from build123d import *

# Parameters (mm, degrees)
CROQUIS1_R              = 31.5
CROQUIS1_R_2            = 1.5
CROQUIS1_R_3            = 2
SALIENTE_EXTRUIR1_DEPTH = 3
CORTAR_EXTRUIR2_DEPTH   = 1.5
CROQUIS4_W              = 15
CROQUIS4_H              = 25
SALIENTE_EXTRUIR2_DEPTH = 3
SALIENTE_EXTRUIR3_DEPTH = 25
CORTAR_EXTRUIR3_DEPTH   = 23
SALIENTE_EXTRUIR4_DEPTH = 5
CORTAR_EXTRUIR4_DEPTH   = 2


with BuildPart() as part:
    # Croquis1 → Saliente-Extruir1 (new body)
    with BuildSketch(Plane.XY):
        with Locations((-43.449193048, 8.207110309)):
            Circle(CROQUIS1_R)
        with Locations((-60.066202406, 24.824119667)):
            Circle(CROQUIS1_R_2, mode=Mode.SUBTRACT)
        with Locations((-26.83218369, 24.824119667)):
            Circle(CROQUIS1_R_2, mode=Mode.SUBTRACT)
        with Locations((-26.83218369, -8.409899049)):
            Circle(CROQUIS1_R_2, mode=Mode.SUBTRACT)
        with Locations((-60.066202406, -8.409899049)):
            Circle(CROQUIS1_R_2, mode=Mode.SUBTRACT)
        with Locations((-43.449193048, 8.207110309)):
            Circle(CROQUIS1_R_3, mode=Mode.SUBTRACT)
    extrude(amount=SALIENTE_EXTRUIR1_DEPTH)

    # Croquis3 → Cortar-Extruir2 (cut)
    with BuildSketch(Plane.XY.offset(3)):
        with BuildLine():
            Line((-41.199193048, 22.957110309), (-40.349193048, 10.457110309))
            Line((-40.349193048, 10.457110309), (-36.699193048, 10.457110309))
            ThreePointArc((-36.699193048, 10.457110309), (-34.449193048, 8.207110309), (-36.699193048, 5.957110309))
            Line((-36.699193048, 5.957110309), (-39.699193048, 5.957110309))
            Line((-39.699193048, 5.957110309), (-41.199193048, -8.542889691))
            ThreePointArc((-41.199193048, -8.542889691), (-43.449193048, -10.792889691), (-45.699193048, -8.542889691))
            Line((-45.699193048, -8.542889691), (-47.199193048, 5.957110309))
            Line((-47.199193048, 5.957110309), (-50.199193048, 5.957110309))
            ThreePointArc((-50.199193048, 5.957110309), (-52.449193048, 8.207110309), (-50.199193048, 10.457110309))
            Line((-50.199193048, 10.457110309), (-46.549193048, 10.457110309))
            Line((-46.549193048, 10.457110309), (-45.699193048, 22.957110309))
            ThreePointArc((-45.699193048, 22.957110309), (-43.449193048, 25.207110309), (-41.199193048, 22.957110309))
        make_face()
    extrude(amount=-CORTAR_EXTRUIR2_DEPTH, mode=Mode.SUBTRACT)

    # Croquis4 → Saliente-Extruir2 (add)
    with BuildSketch(Plane(origin=(0, 0, 0), x_dir=(-1, 0, 0), z_dir=(0, 0, -1))):
        with Locations((43.449193048, 8.207110309)):
            Rectangle(CROQUIS4_W, CROQUIS4_H)
    extrude(amount=SALIENTE_EXTRUIR2_DEPTH)

    # Croquis5 → Saliente-Extruir3 (add)
    with BuildSketch(Plane.XZ.offset(4.292889691)):
        Polygon((-35.949193048, 0), (-32.949193048, 0), (-35.949193048, -3), align=None)
        Polygon((-50.949193048, 0), (-53.949193048, 0), (-50.949193048, -3), align=None)
    extrude(amount=-SALIENTE_EXTRUIR3_DEPTH)

    # Croquis6 → Cortar-Extruir3 (cut)
    with BuildSketch(Plane.XZ.offset(4.292889691)):
        Polygon((-35.949193048, 0), (-50.949193048, 0), (-47.949193048, -3), (-38.949193048, -3), align=None)
    extrude(amount=-CORTAR_EXTRUIR3_DEPTH, mode=Mode.SUBTRACT)

    # Croquis7 → Saliente-Extruir4 (add)
    with BuildSketch(Plane.XZ.offset(4.292889691)):
        Polygon((-39.149193048, -3), (-36.649193048, -0.5), (-36.249193048, -0.5), (-38.749193048, -3), align=None)
        Polygon((-50.249193048, -0.5), (-50.649193048, -0.5), (-48.149193048, -3), (-47.749193048, -3), align=None)
    extrude(amount=SALIENTE_EXTRUIR4_DEPTH)

    # Croquis8 → Cortar-Extruir4 (cut)
    with BuildSketch(Plane(origin=(0, 0, 0), x_dir=(-1, 0, 0), z_dir=(0, 0, -1))):
        Polygon((30.296285305, 24.824119667), (28.564234497, 27.824119667), (25.100132882, 27.824119667), (23.368082075, 24.824119667), (25.100132882, 21.824119667), (28.564234497, 21.824119667), align=None)
        Polygon((63.530304021, 24.824119667), (61.798253213, 27.824119667), (58.334151598, 27.824119667), (56.60210079, 24.824119667), (58.334151598, 21.824119667), (61.798253213, 21.824119667), align=None)
        Polygon((30.296285305, -8.409899049), (28.564234497, -5.409899049), (25.100132882, -5.409899049), (23.368082075, -8.409899049), (25.100132882, -11.409899049), (28.564234497, -11.409899049), align=None)
        Polygon((63.530304021, -8.409899049), (61.798253213, -5.409899049), (58.334151598, -5.409899049), (56.60210079, -8.409899049), (58.334151598, -11.409899049), (61.798253213, -11.409899049), align=None)
    extrude(amount=-CORTAR_EXTRUIR4_DEPTH, mode=Mode.SUBTRACT)


solid = part.part
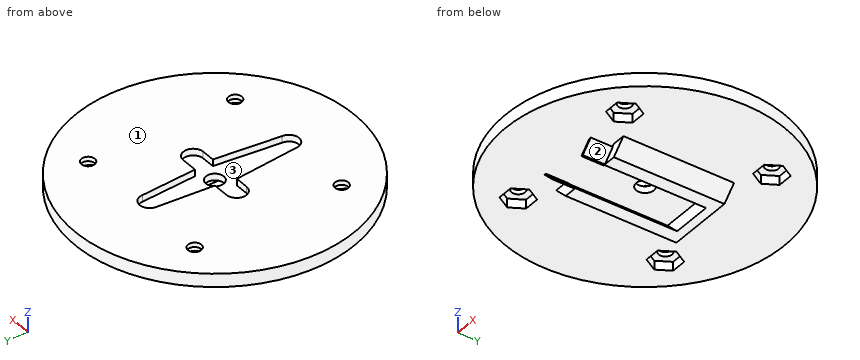
Input: part model. Units: mm. Frame: model coordinates. Face numbers are marked on the shaded views. Give positions to 0.01 mm unless a question says otherwise; leave off trailing zeros. Write each loop counter-clockwise with the first axis right and the second up, starting at its lowest first coordinate (ties: lowest second). Pieces come first, ordered by that corner, then holes. Notation, with made-up numbers: M -20.5,-29 L 28.5,-29 A19 ccw 28.5,-4 Z; hole C -28,54 d2. An arc over 180 degrees is marked long. Write item = value, one per line. Start each with the question number.
1) Cut plane A-A on y = 9. Return the cut outline in (x, z).
2) Cut plane B-B on z = 0.75. Return the cut outline in (x, y), then the cut area to 3 significant figures.
3) Cut plane C-C on x = -44. Return the cut outline in (y, z).
4) Cut plane D-D on y = -0.5. Return the cut outline in (x, z).
5) Draft query along X for the marked faces 1, 2 and 3. Return one class per face: +X half, -X half, draft (parallel to the pull), parting line (faces both ways), or undercut.
6) Material intervals for line 1 along Y through (x, z) = (-24, 0.5); line 2 along X through (y, z) = (23.5, 2.1); line 3 along X through (y, z) = (23, 0.4), sorted ascending. Write a range as [from, to].
7) First-contact query: pin 1 Ø2 at (x, z) = (-33.5, 0) entering from -Y; pin 2 Ø1 at (y, z) = (-10.5, 0.5) entering from -X; pin 3 Ø2 at (x, z) = (-60, 1) entering from -Y; pin 4 Ø2.5 at (x, y) = (-43.45, 8.21) entering from +Z. Flat tips, straight axial feed; report the tip coordinate or a pass-through.
Solved:
q1.outline = M -74.94,0 L -53.95,0 L -50.95,-3 L -47.95,-3 L -50.95,0 L -45.29,0 L -45.29,1.5 L -52.3,1.5 L -52.3,3 L -74.94,3 Z; M -41.61,0 L -35.95,0 L -38.95,-3 L -35.95,-3 L -32.95,0 L -11.96,0 L -11.96,3 L -34.59,3 L -34.59,1.5 L -41.61,1.5 Z
q2.outline = C -43.45,8.21 d63; hole M -63.53,-8.41 L -61.8,-11.41 L -58.33,-11.41 L -56.6,-8.41 L -58.33,-5.41 L -61.8,-5.41 Z; hole M -63.53,24.82 L -61.8,21.82 L -58.33,21.82 L -56.6,24.82 L -58.33,27.82 L -61.8,27.82 Z; hole C -43.45,8.21 d4; hole M -30.3,-8.41 L -28.56,-11.41 L -25.1,-11.41 L -23.37,-8.41 L -25.1,-5.41 L -28.56,-5.41 Z; hole M -30.3,24.82 L -28.56,21.82 L -25.1,21.82 L -23.37,24.82 L -25.1,27.82 L -28.56,27.82 Z
q2.area = 2,980 mm2
q3.outline = M -23.29,0 L 6.28,0 L 6.28,1.5 L -10.72,1.5 L -10.72,3 L -23.29,3 Z; M 10.13,0 L 18.71,0 L 18.71,-3 L 20.71,-3 L 20.71,0 L 39.7,0 L 39.7,3 L 25.14,3 L 25.14,1.5 L 10.13,1.5 Z
q4.outline = M -73.72,0 L -53.95,0 L -50.95,-3 L -47.95,-3 L -50.95,0 L -35.95,0 L -38.95,-3 L -35.95,-3 L -32.95,0 L -13.18,0 L -13.18,3 L -40.37,3 L -40.37,1.5 L -46.53,1.5 L -46.53,3 L -73.72,3 Z
q5.face_1 = draft
q5.face_2 = +X half
q5.face_3 = undercut
q6.line_1 = [-16.57, -9.5], [-7.32, 23.73], [25.92, 32.99]
q6.line_2 = [-70.99, -60.77], [-59.36, -45.63], [-41.27, -27.54], [-26.13, -15.91]
q6.line_3 = [-71.26, -62.48], [-57.66, -29.24], [-24.42, -15.64]
q7.pin_1 = -21.99
q7.pin_2 = -69.15
q7.pin_3 = -19.19
q7.pin_4 = through
